Read the model definition and answer for the solid it produces. Units are mm, in the model's axes. Coordinates: 2 decimals unless noted, no trailing zeros. Loops run counter-clockwise (first coordinate to the right, second up) from the corner with the lowest first, then second, coordinate; pieces in that order, holes last. Notation, with made-up numbers: M 44.25,-21 L 52.25,-21 A26 cw 52.25,13 Z; hole C 55,71.5 d1. An arc over 180 degrees is marked long. One line per item, written item: value. Start each with the question number.
1. The part is cut by section B-B (z = -3). Write down the section's boundary in (x, y).
2. The part is cut by section C-C (x = 11). Write down the section's boundary in (y, z), then the cut area to 3 significant figures.
3. Consider probe 1 along X at (y, z) = (-3.15, 7.5); probe 2 along Y at (x, z) = (-17.5, 23); probe 3 along X at (y, z) = (-3.5, 12). Determine where each line is inside the solid, lowest interval first.
4. The part is cut by section A-A (y = -2.25). Write down the section's boundary in (x, z), then the cut area to 3 significant figures.
```python
from build123d import *

# Parameters (mm, degrees)
F1_DEPTH = 4
F2_SIZE  = 3.5


with BuildPart() as f1:
    # F0 (on Front) → F1 (new body)
    with BuildSketch(Plane.XZ):
        with BuildLine():
            ThreePointArc((25, 19), (23.242641, 23.242641), (19, 25))
            Line((19, 25), (-20, 25))
            ThreePointArc((-20, 25), (-23.535534, 23.535534), (-25, 20))
            Line((-25, 20), (-25, -17))
            ThreePointArc((-25, -17), (-22.656854, -22.656854), (-17, -25))
            Line((-17, -25), (18, -25))
            ThreePointArc((18, -25), (22.949747, -22.949747), (25, -18))
            Line((25, -18), (25, 19))
        make_face()
    extrude(amount=F1_DEPTH)

    # F2
    f2_edges = [f1.edges().sort_by_distance(p)[0] for p in [
        (23.242641, -4, 23.242641),
        (-0.5, -4, 25),
        (-23.535534, -4, 23.535534),
        (-25, -4, 1.5),
        (-22.656854, -4, -22.656854),
        (0.5, -4, -25),
        (22.949747, -4, -22.949747),
        (25, -4, 0.5),
    ]]
    chamfer(f2_edges, length=F2_SIZE)


solid = f1.part
```
Answer block:
1. outline: M -25,-0.5 L -21.5,-4 L 21.5,-4 L 25,-0.5 L 25,0 L -25,0 Z
2. outline: M -4,-21.5 L -0.5,-25 L 0,-25 L 0,25 L -0.5,25 L -4,21.5 Z
2. area: 188 mm2
3. probe 1: x = -22.35 to 22.35
3. probe 2: y = -2.5 to 0
3. probe 3: x = -22 to 22
4. outline: M -23.25,-17 A6.25 ccw -17,-23.25 L 18,-23.25 A5.25 ccw 23.25,-18 L 23.25,19 A4.25 ccw 19,23.25 L -20,23.25 A3.25 ccw -23.25,20 Z
4. area: 2,140 mm2
